The model under review builds one solid part; all positions refer to its coordinate system, in mm. A direction names the side the tool comes from. Round coordinates to 2 decimals unless told otherwise and drop trailing zeros. Write each loop counter-clockwise with the first axis right and the second up, starting at its lowest first coordinate (ties: lowest second). Pieces come first, ordered by that corner, then holes. Notation, with made-up numbers: (-20, 24) - (21, 24) arc R29 ccw to (21, 52) - close; hole circle Ø3 at (16.25, -20). An arc over 180 degrees is marked (long way). Return JSON: item names as keys, results as strings.
from build123d import *
from build123d.topology import SkipClean

# Parameters (mm, degrees)
ESBO_O1_R                  = 21
ESBO_O1_R_2                = 17
RESSALTO_EXTRUS_O1_DEPTH   = 10
RESSALTO_EXTRUS_O2_START   = 4
ESBO_O2_R                  = 21
RESSALTO_EXTRUS_O2_DEPTH   = 4
ESBO_O3_W                  = 15.703263836
ESBO_O3_H                  = 10
CORTE_EXTRUS_O1_DEPTH      = 10
RESSALTO_EXTRUS_O4_START   = -17
ESBO_O8_R                  = 21
ESBO_O8_R_2                = 17
RESSALTO_EXTRUS_O4_DEPTH   = 17
CORTE_EXTRUS_O3_DEPTH      = 27
CORTE_EXTRUS_O3_DEPTH_BACK = 27
ESBO_O12_W                 = 34
ESBO_O12_H                 = 6.5


with BuildPart() as part:
    # Esboço1 → Ressalto-extrusão1 (new body)
    with BuildSketch(Plane.XY):
        Circle(ESBO_O1_R)
        Circle(ESBO_O1_R_2, mode=Mode.SUBTRACT)
    extrude(amount=RESSALTO_EXTRUS_O1_DEPTH)

    # Esboço2 → Ressalto-extrusão2 (add)
    with BuildSketch(Plane(origin=(0, 0, 0), x_dir=(-1, 0, 0), z_dir=(0, 0, -1)).offset(RESSALTO_EXTRUS_O2_START)):
        Circle(ESBO_O2_R)
    extrude(amount=-RESSALTO_EXTRUS_O2_DEPTH)

    # Esboço3 → Corte-extrusão1 (cut)
    with SkipClean():  # the faces are left unmerged after this step: merging them gives an invalid solid
        with BuildSketch(Plane.XY.offset(10)):
            with Locations((-21, 0)):
                Rectangle(ESBO_O3_W, ESBO_O3_H)
        extrude(amount=-CORTE_EXTRUS_O1_DEPTH, mode=Mode.SUBTRACT)

    # Esboço8 → Ressalto-extrusão4 (add)
    with SkipClean():  # the faces are left unmerged after this step: merging them gives an invalid solid
        with BuildSketch(Plane.XY.offset(RESSALTO_EXTRUS_O4_START)):
            with Locations(Location((0, 0, 0), (0, 0, 193.774146998))):
                Circle(ESBO_O8_R)
            Circle(ESBO_O8_R_2, mode=Mode.SUBTRACT)
        extrude(amount=RESSALTO_EXTRUS_O4_DEPTH)
    add(part.part.scale(1), mode=Mode.REPLACE)  # the faces are merged on a copy

    # Esboço12 → Corte-extrusão3 (cut, two sides: drawn at the far end of the back side and taken through both)
    with BuildSketch(Plane(origin=(0, 0, 0), x_dir=(1, 0, 0), z_dir=(0, 1, 0)).offset(-CORTE_EXTRUS_O3_DEPTH_BACK)):
        with Locations((0, 7.25)):
            Rectangle(ESBO_O12_W, ESBO_O12_H)
    extrude(amount=CORTE_EXTRUS_O3_DEPTH + CORTE_EXTRUS_O3_DEPTH_BACK, mode=Mode.SUBTRACT)


solid = part.part
(1) Mouldability with a two-part tool opening along Y and no side actions: class faces 4 (the flat face through (-0.1, 17.5, -10.5)), 5 (the flat face through (-18, -5, 5)) as released by +Y, released by -Y, zero draft, split by the parting line, or undercut.
Filled in:
{"face 4": "zero draft", "face 5": "undercut"}
(2) Add section A-A (x = 0). Write out the cut boundary in (y, z), plus the area to 3 significant figures.
Filled in:
{"outline": "(-21, -17) - (-17, -17) - (-17, -10.5) - (-21, -10.5) - close; (-21, -4) - (21, -4) - (21, 10) - (17, 10) - (17, 0) - (-17, 0) - (-17, 10) - (-21, 10) - close; (17, -17) - (21, -17) - (21, -10.5) - (17, -10.5) - close", "area": "300 mm2"}
(3) Clearance check with flat-ended pins moving along their axes: pin 1 Ø2 at (x, z) = (-17.5, 5) entering from -Y; pin 2 Ø1 at (y, z) = (-3, 7) entering from -X; pin 3 Ø4 at (y, z) = (10, 3.5) entering from -X; pin 4 Ø5 at (y, z) = (15.5, -7) entering from -X. State where each tip first meets the part, or that it passes through.
Filled in:
{"pin 1": "stops at y = -12.99", "pin 2": "stops at x = 16.64", "pin 3": "stops at x = -19.42", "pin 4": "passes through"}
(4) For faces 1 (the flat face through (0, -18, -10.5)), 2 (the cylindrical face through (9.139, 14.334, -13.796)), 3 (the flat face through (-18, 5, 5)), list the 3-axis set-ups (+Z, -Z, +X, -X, +Y, -Y) from which the entire face can be reached by the end or side of a thin tool; tool diameter is ignored.
Filled in:
{"face 1": "+Y, -Y", "face 2": "-Z", "face 3": "+Z, -X"}
(5) Add section B-B (z = -12). Write out the cut boundary in (x, y), plus the area to 3 significant figures.
Filled in:
{"outline": "circle Ø42 at (0, 0); hole circle Ø34 at (0, 0)", "area": "478 mm2"}
(6) Wall thickness on line 1 (Y direction, x = 0, z = -14.5); line 2 (Z direction, x = -6.5, y = -17): over which ranges is each line inside the solid? List them lowest first.
Filled in:
{"line 1": "y = -21 to -17, 17 to 21", "line 2": "z = -17 to -10.5, -4 to 10"}
(7) Add section C-C (y = 7.5). Write out the cut boundary in (x, z), plus the area to 3 significant figures.
Filled in:
{"outline": "(-19.62, -17) - (-15.26, -17) - (-15.26, -10.5) - (-17, -10.5) - (-17, -4) - (17, -4) - (17, -10.5) - (15.26, -10.5) - (15.26, -17) - (19.62, -17) - (19.62, 10) - (15.26, 10) - (15.26, 0) - (-15.26, 0) - (-15.26, 10) - (-19.62, 10) - close", "area": "335 mm2"}
(8) Add section D-D (x = -11). Write out the cut boundary in (y, z).
Filled in:
{"outline": "(-17.89, -17) - (-12.96, -17) - (-12.96, -10.5) - (-17.89, -10.5) - close; (-17.89, -4) - (17.89, -4) - (17.89, 10) - (12.96, 10) - (12.96, 0) - (-12.96, 0) - (-12.96, 10) - (-17.89, 10) - close; (12.96, -17) - (17.89, -17) - (17.89, -10.5) - (12.96, -10.5) - close"}
